CAD build for the part. Positions are in the model's coordinates, mm. A direction names the side the tool comes from. Give positions to 0.01 mm unless a question says otherwise; leave off trailing zeros. Loops run counter-clockwise (first coordinate to the right, second up) from the corner with the lowest first, then second, coordinate; pieces in that order, holes last.
```python
from build123d import *

# Parameters (mm, degrees)
F2_DEPTH = 50.8
F3_START = 76.201
F3_DEPTH = 139.702


with BuildPart() as f2:
    # F0 (on Top) → F2 (new body)
    with BuildSketch(Plane.XY):
        Polygon((50.8, -63.5), (88.9, -63.5), (88.9, 63.5), (-88.9, 63.5), (-88.9, -63.5), (0, -63.5), (0, -76.2), (50.8, -76.2), align=None)
    extrude(amount=F2_DEPTH)

    # F1 (on Front) → F3 (intersect)
    with BuildSketch(Plane.XZ.offset(F3_START)):
        Polygon((-88.9, 50.8), (-88.9, 0), (50.8, 0), (50.8, 21.7714285714), (0, 50.8), align=None)
        Polygon((50.8, 21.7714285714), (50.8, 0), (88.9, 0), align=None)
    extrude(amount=-F3_DEPTH, mode=Mode.INTERSECT)


solid = f2.part
```
1. Saw through at C-C, the plane x = -49. List the corners of the cut face in (y, z), and give its area (3 significant figures).
Responses:
outline: (-63.5, 0) - (63.5, 0) - (63.5, 50.8) - (-63.5, 50.8) - close
area: 6,450 mm2
2. Saw through at D-D, the plane z = 36. List the corners of the cut face in (x, y).
Responses:
outline: (-88.9, -63.5) - (0, -63.5) - (0, -76.2) - (25.9, -76.2) - (25.9, 63.5) - (-88.9, 63.5) - close
3. Drop flat-ended pins along their axis: pin 1 (4 mm diameter, centred on y = 26, z = 32, fed in from +X); pin 2 (3 mm diameter, centred on y = -30, z = 25, fed in from +X) (3 decimals); pin 3 (12 mm diameter, centred on y = -61.5, z = 10.5, fed in from +X) (3 decimals). Give the stop position or say it passes through.
Responses:
pin 1: stops at x = 36.4
pin 2: stops at x = 47.775
pin 3: stops at x = 81.025
4. Saw through at B-B, the plane y = -38.5. List the corners of the cut face in (x, z).
Responses:
outline: (-88.9, 0) - (88.9, 0) - (0, 50.8) - (-88.9, 50.8) - close
5. Saw through at A-A, the plane z = 18. List the corners of the cut face in (x, y), and give its area (3 significant figures).
Responses:
outline: (-88.9, -63.5) - (0, -63.5) - (0, -76.2) - (50.8, -76.2) - (50.8, -63.5) - (57.4, -63.5) - (57.4, 63.5) - (-88.9, 63.5) - close
area: 19,200 mm2
6. Probe line 1 along Y through (x, z) = (-72.5, 13.5); line 2 along X through (y, z) = (-58.5, 37.5) (3 decimals); line 3 along X through (y, z) = (39, 40). List the from-to ranges inside material, lowest first.
Responses:
line 1: y = -63.5 to 63.5
line 2: x = -88.9 to 23.275
line 3: x = -88.9 to 18.9
7. Tool access for faces 1 (the face through (0, -70, 25)), 2 (the face through (-1, -5, 0)), 3 (the face through (65, -63.5, 8)): list every direction of +Z, -Z, +X, -X, +Y, -Y with a clear straight run to the whole face (end or side of a thin tool).
Responses:
face 1: +Z, -Z, -X, -Y
face 2: -Z, +X, -X, +Y, -Y
face 3: +Z, -Z, +X, -Y
